from build123d import *

# Parameters (mm, degrees)
F1_DEPTH  = 100
F3_DEPTH  = 10
F8_DEPTH  = 3
F10_DEPTH = 25
F12_DEPTH = 10
F14_R     = 14
F14_R_2   = 7.5
F15_DEPTH = 8
F16_R     = 7.5
F17_DEPTH = 25
F19_D     = 13


with BuildPart() as f1:
    # F0 (on Front) → F1 (new body)
    with BuildSketch(Plane.XZ):
        Polygon((50, 0), (0, 0), (0, -30), (14, -30), (14, -34.8), (36, -34.8), (36, -30), (50, -30), align=None)
    extrude(amount=F1_DEPTH)

    # F2 (on face) → F3 (join)
    with BuildSketch(Plane(origin=(0, 0, 0), x_dir=(0, -1, 0), z_dir=(-1, 0, 0))):
        with BuildLine():
            Line((43.2649507991, 54.3428379122), (0, 0))
            Line((0, 0), (100, 0))
            Line((100, 0), (100, 45))
            ThreePointArc((100, 45), (95.6066017178, 55.6066017178), (85, 60))
            Line((85, 60), (55, 60))
            ThreePointArc((55, 60), (48.4862671487, 58.5118941804), (43.2649507991, 54.3428379122))
        make_face()
    extrude(amount=-F3_DEPTH)


with BuildPart() as f5_1:
    # F5: instance of F1
    add(f1.part.mirror(Plane(origin=(22.8108581436, -50, -11.9144915301), x_dir=(1, 0, 0), z_dir=(0, 1, 0))))

    # F7 (on face) → F8 (join)
    with BuildSketch(Plane.YZ.offset(10)):
        with BuildLine():
            ThreePointArc((-15, 30), (-4.3933982822, 34.3933982822), (0, 45))
            ThreePointArc((0, 45), (-4.3933982822, 55.6066017178), (-15, 60))
            Line((-15, 60), (-45, 60))
            ThreePointArc((-45, 60), (-51.5137328513, 58.5118941804), (-56.7350492009, 54.3428379122))
            ThreePointArc((-56.7350492009, 54.3428379122), (-58.5118941804, 38.4862671487), (-45, 30))
            Line((-45, 30), (-15, 30))
        make_face()
        with BuildLine():
            ThreePointArc((-45, 35), (-55, 45), (-45, 55))
            Line((-45, 55), (-15, 55))
            ThreePointArc((-15, 55), (-5, 45), (-15, 35))
            Line((-15, 35), (-45, 35))
        make_face(mode=Mode.SUBTRACT)
    extrude(amount=F8_DEPTH)

    # F9 (on face) → F10 (cut)
    with BuildSketch(Plane.YZ.offset(10)):
        with BuildLine():
            Line((-15, 55), (-45, 55))
            ThreePointArc((-45, 55), (-55, 45), (-45, 35))
            Line((-45, 35), (-15, 35))
            ThreePointArc((-15, 35), (-5, 45), (-15, 55))
        make_face()
    extrude(amount=-F10_DEPTH, mode=Mode.SUBTRACT)

    # F11 (on face) → F12 (join)
    with BuildSketch(Plane.XY):
        with BuildLine():
            Line((50, -50), (50, -79))
            Line((50, -79), (90.1775700039, -63.0074120737))
            ThreePointArc((90.1775700039, -63.0074120737), (99, -50), (90.1775700039, -36.9925879263))
            Line((90.1775700039, -36.9925879263), (50, -21))
            Line((50, -21), (50, -50))
        make_face()
    extrude(amount=-F12_DEPTH)

    # F14 (on mid) → F15 (join, symmetric)
    with BuildSketch(Plane(origin=(0, 0, -5), x_dir=(1, 0, 0), z_dir=(0, 0, -1))):
        with Locations((85, 50)):
            Circle(F14_R)
        with Locations((85, 50)):
            Circle(F14_R_2, mode=Mode.SUBTRACT)
    extrude(amount=F15_DEPTH, both=True)

    # F16 (on face) → F17 (cut)
    with BuildSketch(Plane.XY):
        with Locations((85, -50)):
            Circle(F16_R)
    extrude(amount=-F17_DEPTH, mode=Mode.SUBTRACT)

    # F19 (through all)
    with Locations(Plane.XZ.offset(100)):
        with Locations((25, -18.8)):
            Hole(F19_D / 2)


solid = f5_1.part
Read the model definition and answer for the solid it produces. Units are mm, in the model's axes. A direction names the side the tool comes from. Give positions to 0.01 mm unless a question says otherwise; leave off trailing zeros. Loops run counter-clockwise (first coordinate to the right, second up) from the corner with the lowest first, then second, coordinate; pieces in that order, holes last. Notation, with made-up numbers: (79.5, 84) - (84.5, 84) arc R21 cw to (84.5, 121) - close; hole circle Ø3 at (-27, -22.75). An arc over 180 degrees is marked (long way). Answer as CSV lines item,"result". Start each with the question number.
1) Find section B-B (z = -18.8). Write down the section's boundary in (x, y).
2) Straight lines are drawn through the part: L1, parallel to X at y = -50, z = 1.45; L2, parallel to Z at x = 5, y = -32.5; L3, parallel to X at y = -50, z = -11.6. For each, find the intervals that lie inside material, in ascending order. Write a range as from..to.
3) Determine the mould class of faces 1 (the face through (7, -51, -30)), 2 (the face through (36, -51, -32)), 3 (the face through (6, -30, 35)) for opening direction Z: released by +Z, released by -Z, zero draft, split by the parting line, or undercut.
4) Find section A-A (x = 25). Write down the section's boundary in (y, z), then the cut area to 3 significant figures.
5) Which of the six approach directions +Z, -Z, +X, -X, +Y, -Y give full straight-line access (tool end or side, diameter ignored) to faces 4 (the face through (11, -30, 30)), 5 (the face through (43, -51, -30)), 6 (the face through (91, -44, 3))?
6) Each of these flat-tipped pins is pushed along its axis until it touches: pin 1 Ø8 at (x, z) = (14, -21.5) entering from +Y; pin 2 Ø2.5 at (y, z) = (-47.5, -31.5) entering from +X; pin 3 Ø1 at (x, y) = (47.5, -53) entering from +Z; pin 4 Ø0.9 at (x, y) = (11, -29.5) entering from -Z. Where does it stop, or does it pass through?
7) Find section C-C (y = -84.5). Write down the section's boundary in (x, z).
8) Find section D-D (x = 85). Write down the section's boundary in (y, z).
Findings below:
1,outline,"(0, -100) - (18.5, -100) - (18.5, 0) - (0, 0) - close; (31.5, -100) - (50, -100) - (50, 0) - (31.5, 0) - close"
2,L1,"0..10, 71..77.5, 92.5..99"
2,L2,"-30..35, 55..60"
2,L3,"0..50, 71..77.5, 92.5..99"
3,face 1,"released by -Z"
3,face 2,"zero draft"
3,face 3,"undercut"
4,outline,"(-100, -34.8) - (0, -34.8) - (0, -25.3) - (-100, -25.3) - close; (-100, -12.3) - (0, -12.3) - (0, 0) - (-100, 0) - close"
4,area,"2,180 mm^2"
5,face 4,"+X, +Y, -Y"
5,face 5,"-Z, +X, +Y, -Y"
5,face 6,"+Z, +X, +Y, -Y"
6,pin 1,"y = 0"
6,pin 2,"x = 36"
6,pin 3,"z = 0"
6,pin 4,"z = -30"
7,outline,"(0, -30) - (14, -30) - (14, -34.8) - (36, -34.8) - (36, -30) - (50, -30) - (50, 0) - (10, 0) - (10, 19.47) - (0, 19.47) - close; hole circle Ø13 at (25, -18.8)"
8,outline,"(-65.07, -10) - (-64, -10) - (-64, -13) - (-57.5, -13) - (-57.5, 3) - (-64, 3) - (-64, 0) - (-65.07, 0) - close; (-42.5, -13) - (-36, -13) - (-36, -10) - (-34.93, -10) - (-34.93, 0) - (-36, 0) - (-36, 3) - (-42.5, 3) - close"
